Geometry check sheet. Reference: the model listing, model coordinates, mm. A direction names the side the tool comes from. Round coordinates to 2 decimals unless told otherwise and drop trailing zeros. Write each loop counter-clockwise with the first axis right and the second up, starting at its lowest first coordinate (ties: lowest second). Pieces come first, ordered by that corner, then holes.
Item 1: Cross-section at C-C (y = 5). Enter the section's corners in (x, z), then the cut area to 3 significant figures.
Item 2: Cross-section at D-D (z = 0). Enter the section's corners in (x, y).
Item 3: Depth check by flat-ended pin: P1, Ø1, axis at y = 1.5, z = -4.5, coming from the +X side; P2, Ø6, axis at x = -0.5, z = 2.5, coming from the +Y side; P3, Ø2, axis at x = 0, y = 5, coming from the +Z side. Enter the tip coordinate at first touch or a pass-through.
Item 4: Cross-section at A-A (z = 8). Enter the section's corners in (x, y).
Item 5: Draft check along X on faces 4 (the face through (5.1, 5.1, -13.2)), 5 (the face through (1.802, 4.93, 5.723)), 6 (the face through (10.65, 4.93, -2.45)), 7 (the face through (8, 5, -16)). Enter one of: pulls with the +X half, pulls with the -X half, needs draft (parallel to the pull), parting line crosses it, or undercut.
Item 6: Scan lines: probe 1 along X at (y, z) = (2.5, -7.75); probe 2 along Z at (x, y) = (0, 3.75); probe 3 along X at (y, z) = (9.5, -10.5). Record each from-to range of solid material in increasing order.
Item 7: Access from +Z, -Z, +X, -X, +Y, -Y to the whole of each face (thin tool, end or side, straight path). Record for faces 1 (the face through (2, 10, -7)), 2 (the face through (-5.05, 4.93, -15.64)), 3 (the face through (-0.21, 6.62, 8.42)).
Item 8: Cross-section at B-B (x = -11). Enter the section's corners in (y, z), then the cut area to 3 significant figures.
from build123d import *

# Parameters (mm, degrees)
CROQUIS1_R              = 10
CROQUIS1_R_2            = 6
SALIENTE_EXTRUIR1_DEPTH = 10
CROQUIS2_R              = 4
CORTAR_EXTRUIR1_DEPTH   = 10
CHAFL_N1_DEPTH          = 10
CROQUIS3_W              = 5
CROQUIS3_H              = 2
SALIENTE_EXTRUIR2_DEPTH = 10
CROQUIS4_R              = 1.635125
CORTAR_EXTRUIR2_DEPTH   = 10
REDONDEO2_R             = 4


with BuildPart() as part:
    # Croquis1 → Saliente-Extruir1 (new body)
    # profile 1 of 2: a face of its own
    with BuildSketch(Plane(origin=(0, 0, 0), x_dir=(1, 0, 0), z_dir=(0, 1, 0))):
        Circle(CROQUIS1_R)
        with Locations(Location((0, 0, 0), (0, 0, 270))):
            Circle(CROQUIS1_R_2, mode=Mode.SUBTRACT)
    # profile 2 of 2: a face of its own
    with BuildSketch(Plane(origin=(0, 0, 0), x_dir=(1, 0, 0), z_dir=(0, 1, 0))):
        with BuildLine():
            Line((-14, 16), (-4.582575695, 16))
            ThreePointArc((-4.582575695, 16), (0, 13), (4.582575695, 16))
            Line((4.582575695, 16), (14, 16))
            Line((14, 16), (14, 6))
            Line((14, 6), (-14, 6))
            Line((-14, 6), (-14, 16))
        make_face()
    extrude(amount=SALIENTE_EXTRUIR1_DEPTH)

    # Croquis2 → Cortar-Extruir1 (cut)
    with BuildSketch(Plane(origin=(0, 10, 0), x_dir=(1, 0, 0), z_dir=(0, 1, 0))):
        with Locations(Location((-7.5, 10, 0), (0, 0, 270))):
            Circle(CROQUIS2_R)
        with Locations(Location((7.5, 10, 0), (0, 0, 270))):
            Circle(CROQUIS2_R)
    extrude(amount=-CORTAR_EXTRUIR1_DEPTH, mode=Mode.SUBTRACT)

    # Chaflán1: read off the stored shape, not the designer's step
    # Chaflán1 outline → Chaflán1 (add)
    with BuildSketch(Plane(origin=(0, 0, 0), x_dir=(1, 0, 0), z_dir=(0, 1, 0))):
        with BuildLine():
            ThreePointArc((8, 6), (9.633249581, 2.68337521), (9.949874371, -1))
            Line((9.949874371, -1), (11.371284996, 6))
            Line((11.371284996, 6), (8, 6))
        make_face()
        with BuildLine():
            Line((-11.371284996, 6), (-9.949874371, -1))
            ThreePointArc((-9.949874371, -1), (-9.633249581, 2.68337521), (-8, 6))
            Line((-8, 6), (-11.371284996, 6))
        make_face()
    extrude(amount=CHAFL_N1_DEPTH)

    # Croquis3 → Saliente-Extruir2 (add)
    with BuildSketch(Plane(origin=(0, 0, 0), x_dir=(1, 0, 0), z_dir=(0, 1, 0))):
        with Locations((0, -10)):
            Rectangle(CROQUIS3_W, CROQUIS3_H)
    extrude(amount=SALIENTE_EXTRUIR2_DEPTH)

    # Croquis4 → Cortar-Extruir2 (cut)
    with BuildSketch(Plane.XY.offset(11)):
        with Locations((0, 5)):
            Circle(CROQUIS4_R)
    extrude(amount=-CORTAR_EXTRUIR2_DEPTH, mode=Mode.SUBTRACT)

    # Redondeo2
    # the kernel refuses this fillet: 4 mm, written as the material it adds along each edge
    with BuildSketch(Plane(origin=(2.5, 10, 9.682458366), x_dir=(0, 0, 1), z_dir=(0, -1, 0))) as redondeo2_piece_1:
        with BuildLine():
            CenterArc((2.878230853, -3.68296744), REDONDEO2_R, 112.965221116, 40.826178459)
            Line((-0.710537495, -1.916405314), (-0.782312862, -1.881074072))
            ThreePointArc((-0.782312862, -1.881074072), (-0.381189036, -0.948592301), (-0.077459667, 0.02))
            Line((-0.077459667, 0.02), (0, 0.08))
            ThreePointArc((0, 0.08), (0.658770817, 0.08), (1.28632785, 0.073659349))
            Line((1.28632785, 0.073659349), (1.317541634, 0))
        make_face()
    extrude(amount=10)
    with BuildSketch(Plane(origin=(-2.5, 10, 9.682458366), x_dir=(-0.9376279565956984, 0, -0.3476403529657844), z_dir=(0, -1, 0))) as redondeo2_piece_2:
        with BuildLine():
            CenterArc((2.452664045, -3.979057814), REDONDEO2_R, 95.865544119, 40.826178459)
            Line((-0.458030639, -1.23536387), (-0.516244533, -1.180489992))
            ThreePointArc((-0.516244533, -1.180489992), (-0.304025556, -0.589870707), (-0.075010237, 0.027811228))
            Line((-0.075010237, 0.027811228), (0.008175547, 0.079581156))
            ThreePointArc((0.008175547, 0.079581156), (1.021943352, 0.027644534), (2.035711158, 0.079581156))
            Line((2.035711158, 0.079581156), (2.043886705, 0))
        make_face()
    extrude(amount=10)
    # the kernel refuses this fillet: 4 mm, written as the material it takes off along each edge
    with BuildSketch(Plane(origin=(4.582575695, -5.314070594, -16), x_dir=(-0.5401558180759948, 0, 0.8415650255319863), z_dir=(0, 1, 0))) as redondeo2_2_piece_1:
        with BuildLine():
            CenterArc((2.218089643, 3.949477654), REDONDEO2_R, 212.694246687, 48.189685104)
            Line((-1.14817046, 1.788854382), (-1.215495662, 1.745641917))
            Line((-1.215495662, 1.745641917), (-0.067325202, -0.043212465))
            Line((-0.067325202, -0.043212465), (0.012674798, -0.078989553))
            ThreePointArc((0.012674798, -0.078989553), (0.792174872, -0.016847068), (1.571674947, -0.078989553))
            Line((1.571674947, -0.078989553), (1.584349745, 0))
        make_face()
    extrude(amount=20.628141188, mode=Mode.SUBTRACT)
    with BuildSketch(Plane(origin=(14, -10, -16), x_dir=(-1, 0, 0), z_dir=(0, 1, 0)), Plane(origin=(-14, -10, -16), x_dir=(0, 0, 1), z_dir=(0, 1, 0))) as redondeo2_2_piece_2:
        with BuildLine():
            CenterArc((REDONDEO2_R, REDONDEO2_R), REDONDEO2_R, 180, 90)
            Line((0, REDONDEO2_R), (-REDONDEO2_R * 0.02, REDONDEO2_R))
            Line((-REDONDEO2_R * 0.02, REDONDEO2_R), (-REDONDEO2_R * 0.02, -REDONDEO2_R * 0.02))
            Line((-REDONDEO2_R * 0.02, -REDONDEO2_R * 0.02), (REDONDEO2_R, -REDONDEO2_R * 0.02))
            Line((REDONDEO2_R, -REDONDEO2_R * 0.02), (REDONDEO2_R, 0))
        make_face()
    extrude(amount=30, mode=Mode.SUBTRACT)
    with BuildSketch(Plane(origin=(-4.582575695, -5.314070594, -16), x_dir=(-1, 0, 0), z_dir=(0, 1, 0))) as redondeo2_2_piece_3:
        with BuildLine():
            CenterArc((2.125628238, 4), REDONDEO2_R, 221.810314896, 48.189685104)
            Line((-0.855795732, 1.333333333), (-0.915424212, 1.28))
            ThreePointArc((-0.915424212, 1.28), (-0.442075769, 0.657566625), (-0.073321211, -0.032))
            Line((-0.073321211, -0.032), (0, -0.08))
            Line((0, -0.08), (2.125628238, -0.08))
            Line((2.125628238, -0.08), (2.125628238, 0))
        make_face()
    extrude(amount=20.628141188, mode=Mode.SUBTRACT)
    with BuildSketch(Plane(origin=(14, -9.394006553, -6), x_dir=(0, 0, -1), z_dir=(0, 1, 0))) as redondeo2_2_piece_4:
        with BuildLine():
            CenterArc((3.757602621, 4), REDONDEO2_R, 200.048853319, 69.951146681)
            Line((0, 2.628715004), (-0.075152052, 2.601289304))
            ThreePointArc((-0.075152052, 2.601289304), (-0.08, 1.314357502), (-0.08, 0))
            Line((-0.08, 0), (0, -0.08))
            Line((0, -0.08), (3.757602621, -0.08))
            Line((3.757602621, -0.08), (3.757602621, 0))
        make_face()
    extrude(amount=28.788013107, mode=Mode.SUBTRACT)
    with BuildSketch(Plane(origin=(-14, -9.394006553, -6), x_dir=(1, 0, 0), z_dir=(0, 1, 0))) as redondeo2_2_piece_5:
        with BuildLine():
            CenterArc((4, 3.757602621), REDONDEO2_R, 180, 69.951146681)
            Line((0, 3.757602621), (-0.08, 3.757602621))
            Line((-0.08, 3.757602621), (-0.08, 0))
            Line((-0.08, 0), (0, -0.08))
            ThreePointArc((0, -0.08), (1.314357502, -0.08), (2.601289304, -0.075152052))
            Line((2.601289304, -0.075152052), (2.628715004, 0))
        make_face()
    extrude(amount=28.788013107, mode=Mode.SUBTRACT)


solid = part.part
Resolved:
1. outline: (-14, -12) arc R4 ccw to (-10, -16) - (-6.71, -16) arc R4 ccw to (-3.73, -14.67) arc R5 cw to (3.73, -14.67) arc R4 ccw to (6.71, -16) - (10, -16) arc R4 ccw to (14, -12) - (14, -9.76) arc R4 ccw to (11.37, -6) - (9.95, 1) arc R10 ccw to (4.42, 8.97) arc R4 cw to (2.5, 11) - (1.64, 11) - (1.64, 5.77) arc R6 cw (long way) to (-1.64, 5.77) - (-1.64, 11) - (-2.5, 11) arc R4 cw to (-4.42, 8.97) arc R10 ccw to (-9.95, 1) - (-11.37, -6) arc R4 ccw to (-14, -9.76) - close; hole circle Ø8 at (-7.5, -10); hole circle Ø8 at (7.5, -10)
1. area: 310 mm2
2. outline: (-10.15, 0) - (-6, 0) - (-6, 10) - (-10.15, 10) - close; (6, 0) - (10.15, 0) - (10.15, 10) - (6, 10) - close
3. P1: stops at x = 11.17
3. P2: passes through
3. P3: stops at z = -5.92
4. outline: (-6, 0) - (6, 0) - (6, 10) - (-6, 10) - close; hole circle Ø3.27 at (0, 5)
5. face 4: undercut
5. face 5: undercut
5. face 6: pulls with the +X half
5. face 7: needs draft
6. probe 1: x = -13.46 to -10.81, -4.19 to 4.19, 10.81 to 13.46
6. probe 2: z = -13 to -6
6. probe 3: x = -14 to -11.47, -3.53 to 3.53, 11.47 to 14
7. face 1: +Z, -Z, +X, -X, +Y
7. face 2: -Z, +Y, -Y
7. face 3: +Z
8. outline: (0, -15.87) - (10, -15.87) - (10, -11.94) - (0, -11.94) - close; (0, -8.06) - (10, -8.06) - (10, -4.17) - (0, -4.17) - close
8. area: 78.3 mm2
